```python
from build123d import *

# Parameters (mm, degrees)
F0_W           = 82.55
F0_H           = 35.56
F1_DEPTH       = 95.25
F3_D           = 6.35
F3_DEPTH       = 19.05
F3_TIP         = 1.9077324654
F5_D           = 6.35
F5_DEPTH       = 19.05
F5_TIP         = 1.9077324654
F7_DEPTH       = 82.55
F9_D           = 6.35
F9_CBORE_D     = 12.7
F9_CBORE_DEPTH = 3.175
F10_R          = 6.35
F11_R          = 3.175


with BuildPart() as f1:
    # F0 (on Front) → F1 (new body)
    with BuildSketch(Plane.XZ):
        with Locations((41.275, 17.78)):
            Rectangle(F0_W, F0_H)
    extrude(amount=F1_DEPTH)

    # F3
    with Locations(Plane.XZ.offset(95.25)):
        with Locations((7.9248, 25.4), (74.5998, 25.4)):
            Hole(F3_D / 2, depth=F3_DEPTH)
            with Locations((0, 0, -(F3_DEPTH + F3_TIP / 2))):  # 118° drill point
                Cone(0, F3_D / 2, F3_TIP, mode=Mode.SUBTRACT)

    # F5
    with Locations(Plane(origin=(0, 0, 0), x_dir=(-1, 0, 0), z_dir=(0, 1, 0))):
        with Locations((-12.7, 17.78), (-69.85, 17.78)):
            Hole(F5_D / 2, depth=F5_DEPTH)
            with Locations((0, 0, -(F5_DEPTH + F5_TIP / 2))):  # 118° drill point
                Cone(0, F5_D / 2, F5_TIP, mode=Mode.SUBTRACT)

    # F6 (on Right) → F7 (join)
    with BuildSketch(Plane.YZ):
        with BuildLine():
            Line((0, -9.525), (0, 0))
            Line((0, 0), (-9.525, 0))
            Line((-9.525, 0), (-95.25, 0))
            Line((-95.25, 0), (-95.25, -9.525))
            Line((-95.25, -9.525), (-15.875, -9.525))
            ThreePointArc((-15.875, -9.525), (-11.3848719395, -11.3848719395), (-9.525, -15.875))
            Line((-9.525, -15.875), (-9.525, -52.6542))
            Line((-9.525, -52.6542), (0, -52.6542))
            Line((0, -52.6542), (0, -9.525))
        make_face()
    extrude(amount=F7_DEPTH)

    # F9 (through all)
    with Locations(Plane.XZ.offset(9.525)):
        with Locations((14.732, -39.9542), (67.818, -39.9542)):
            CounterBoreHole(F9_D / 2, F9_CBORE_D / 2, F9_CBORE_DEPTH)

    # F10
    f10_edges = [f1.edges().sort_by_distance(p)[0] for p in [
        (0, -4.7625, -52.6542),
        (82.55, -4.7625, -52.6542),
    ]]
    fillet(f10_edges, radius=F10_R)

    # F11
    f11_edges = [f1.edges().sort_by_distance(p)[0] for p in [
        (82.55, -95.25, 13.0175),
        (41.275, -95.25, -9.525),
        (0, -95.25, 13.0175),
        (0, -55.5625, -9.525),
        (82.55, -47.625, 35.56),
        (41.275, -95.25, 35.56),
        (0, -47.625, 35.56),
        (41.275, 0, 35.56),
        (0, 0, -5.3721),
    ]]
    fillet(f11_edges, radius=F11_R)


solid = f1.part
```
Check sheet for the modelled part. Datum: model origin and axes. Units: mm. A direction names the side the tool comes from. Round coordinates to 2 decimals unless told otherwise and drop trailing zeros. Order: outer loops, then holes, each group sorted by start corner. A loop starts at its lowest first (then second) coordinate and runs counter-clockwise, first axis right, second up. Notation, with made-up numbers: (63, 14) - (74, 14) arc R17 ccw to (74, 30) - close; hole circle Ø5 at (78, -0.75). An arc over 180 degrees is marked (long way). Answer as CSV lines item,"result". Start each with the question number.
1) Section check C-C (x = 34). Record the cut outline in (y, z) (3 decimals).
2) Scan lines: probe 1 along Y at (x, z) = (53.5, -32) (3 decimals); probe 2 along Z at (x, y) = (77.5, -21) (3 decimals); probe 3 along Y at (x, z) = (71.5, 25). Record each from-to range of solid material in increasing order.
3) Depth check by flat-ended pin: pin 1 (8.5 mm diameter, centred on x = 12.7, z = 17.78, fed in from +Y); pin 2 (5.5 mm diameter, centred on x = 69.85, z = 17.78, fed in from +Y); pin 3 (2 mm diameter, centred on x = 74, y = -71, fed in from -Z) (3 decimals); pin 4 (6.5 mm diameter, centred on x = 16, z = -37.5, fed in from -Y). Enter the tip coordinate at first touch or a pass-through.
4) Draft check along X on faces 1 (the face through (7.853, -74.624, 25.947)), 2 (the face through (41, -9.525, -32)), 3 (the face through (80.739, -4.74, -50.745)), 4 (the face through (0, -48, 11)). Enter one of: +X half, -X half, draft (parallel to the pull), parting line (faces both ways), or undercut.
5) Section check A-A (y = -83.5). Record the cut outline in (x, z) (3 decimals), then the cut area to 3 significant figures.
6) Section check D-D (y = -47). Record the cut outline in (x, z) (3 decimals), then the cut area to 3 significant figures.
7) Tool access check on faces 5 (the face through (81.645, -54.508, -8.57)), 6 (the face through (81.6, -94.34, 13.29)), 7 (the face through (8.338, -85.592, 28.548)), 8 (the face through (41, -55, -9.525)), 9 (the face through (0.9, -48.2, 34.6)). Record the directions out of +Z, -Z, +X, -X, +Y, -Y that give a thin tool (end or side, any length) a straight path to the whole face; none if there is none.
8) Section check B-B (z = -25). Record the cut outline in (x, y) (3 decimals).
Determined:
1,outline,"(-95.25, -6.35) arc R3.175 ccw to (-92.075, -9.525) - (-15.875, -9.525) arc R6.35 cw to (-9.525, -15.875) - (-9.525, -49.479) arc R3.175 ccw to (-6.35, -52.654) - (-3.175, -52.654) arc R3.175 ccw to (0, -49.479) - (0, 32.385) arc R3.175 ccw to (-3.175, 35.56) - (-92.075, 35.56) arc R3.175 ccw to (-95.25, 32.385) - close"
2,probe 1,"-9.525 to 0"
2,probe 2,"-9.525 to 35.56"
2,probe 3,"-76.17 to 0"
3,pin 1,"y = 0"
3,pin 2,"y = -19.31"
3,pin 3,"z = -9.525"
3,pin 4,"y = -6.35"
4,face 1,"undercut"
4,face 2,"draft"
4,face 3,"+X half"
4,face 4,"-X half"
5,outline,"(0, -6.35) arc R3.175 ccw to (3.175, -9.525) - (79.375, -9.525) arc R3.175 ccw to (82.55, -6.35) - (82.55, 32.385) arc R3.175 ccw to (79.375, 35.56) - (3.175, 35.56) arc R3.175 ccw to (0, 32.385) - close; hole circle Ø6.35 at (7.925, 25.4); hole circle Ø6.35 at (74.6, 25.4)"
5,area,"3,650 mm^2"
6,outline,"(0, -6.35) arc R3.175 ccw to (3.175, -9.525) - (79.375, -9.525) arc R3.175 ccw to (82.55, -6.35) - (82.55, 32.385) arc R3.175 ccw to (79.375, 35.56) - (3.175, 35.56) arc R3.175 ccw to (0, 32.385) - close"
6,area,"3,710 mm^2"
7,face 5,"-Z, +X, -Y"
7,face 6,"+Z, -Z, +X, -Y"
7,face 7,"-Y"
7,face 8,"-Z, +X, -X, -Y"
7,face 9,"+Z, -X, +Y, -Y"
8,outline,"(0, -6.35) arc R3.175 ccw to (3.175, -9.525) - (79.375, -9.525) arc R3.175 ccw to (82.55, -6.35) - (82.55, -3.175) arc R3.175 ccw to (79.375, 0) - (3.175, 0) arc R3.175 ccw to (0, -3.175) - close"
